from build123d import *

# Parameters (mm, degrees)
F0_W     = 10
F0_H     = 120
F1_DEPTH = 40
F2_SIZE  = 10
F4_DEPTH = 40
F5_R     = 15


with BuildPart() as f1:
    # F0 (on Front) → F1 (new body)
    with BuildSketch(Plane.XZ):
        with Locations((5, 60)):
            Rectangle(F0_W, F0_H)
    extrude(amount=-F1_DEPTH)

    # F2
    f2_edges = [f1.edges().sort_by_distance(p)[0] for p in [
        (5, 0, 120),
        (5, 40, 120),
    ]]
    chamfer(f2_edges, length=F2_SIZE)

    # F3 (on face) → F4 (cut, through all)
    with BuildSketch(Plane.XZ):
        with BuildLine():
            ThreePointArc((10, 78.97916), (4.9999989609, 55), (10, 31.02084))
            Line((10, 31.02084), (10, 78.97916))
        make_face()
    extrude(amount=-F4_DEPTH, mode=Mode.SUBTRACT)

    # F5
    f5_edges = [f1.edges().sort_by_distance(p)[0] for p in [
        (10, 20, 31.02084),
        (10, 20, 78.97916),
    ]]
    fillet(f5_edges, radius=F5_R)


solid = f1.part
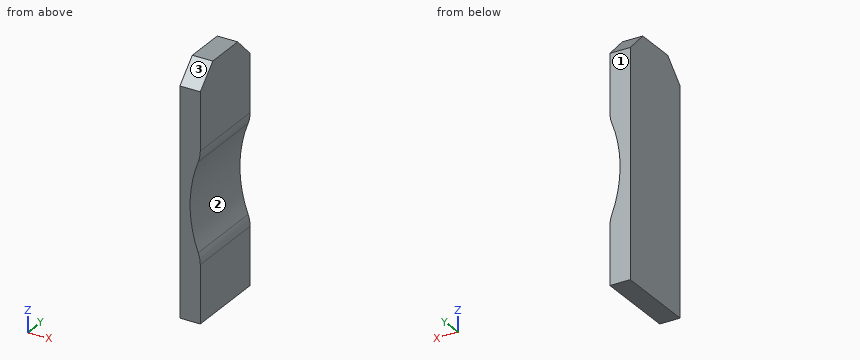
Could you check a few things on this model? Use its own coordinates, in mm. Face numbers are marked on the shaded views. Round coordinates to 2 decimals unless told otherwise and drop trailing zeros. Loops run counter-clockwise (first coordinate to the right, second up) from the corner with the lowest first, then second, coordinate; pieces in that order, holes last. Notation, with made-up numbers: (3, -36.75) -> (17, -36.75) arc R32 cw to (17, -0.75) -> close; hole circle Ø5 at (-14.5, 6.25). An arc over 180 degrees is marked (long way). Use CSV: the item, a comma, the result in double quotes.
(1) Suppose I cut it at D-D on z = 31. Write out the boundary of the cut face in (x, y).
Return value:
outline,"(0, 0) -> (9.71, 0) -> (9.71, 40) -> (0, 40) -> close"
(2) If we mould it in two halves opening along Z, with no side actions, what happens to the marked faces 1, 2 and 3? For each: +Z half, -Z half, draft (parallel to the pull), parting line (faces both ways), or undercut.
Return value:
face 1,"draft"
face 2,"undercut"
face 3,"+Z half"
(3) If I drill on probe 1 along X at (y, z) = (19, 76.5); probe 2 along X at (y, z) = (25.5, 34.5); probe 3 along Z at (x, y) = (2.5, 7), over which ranges is the centre line in solid material (lowest first)? Write a range as [from, to].
Return value:
probe 1,"x = [0, 8.98]"
probe 2,"x = [0, 8.61]"
probe 3,"z = [0, 117]"
(4) Suppose I cut it at B-B on x = 7. Write out the boundary of the cut face in (y, z), plus the area to 3 significant figures.
Return value:
outline,"(0, 0) -> (40, 0) -> (40, 39.64) -> (0, 39.64) -> close; (0, 70.36) -> (40, 70.36) -> (40, 110) -> (30, 120) -> (10, 120) -> (0, 110) -> close"
area,"3,470 mm²"
(5) Will this pin go through, and if not, where does the flat tip stop? pin 1 Ø5 at (y, z) = (30, 57) entering from +X.
Return value:
pin 1,"stops at x = 5.17"
(6) Suppose I cut it at A-A on y = 31.5. Write out the boundary of the cut face in (x, z).
Return value:
outline,"(0, 0) -> (10, 0) -> (10, 28.07) arc R15 ccw to (9, 33.46) arc R60 cw to (9, 76.54) arc R15 ccw to (10, 81.93) -> (10, 118.5) -> (0, 118.5) -> close"
(7) Suppose I cut it at C-C on y = 36.5. Write out the boundary of the cut face in (x, z), plus the area to 3 significant figures.
Return value:
outline,"(0, 0) -> (10, 0) -> (10, 28.07) arc R15 ccw to (9, 33.46) arc R60 cw to (9, 76.54) arc R15 ccw to (10, 81.93) -> (10, 113.5) -> (0, 113.5) -> close"
area,"973 mm²"
